```python
from build123d import *

# Parameters (mm, degrees)
SKETCH046_R     = 2.5
PAD023_DEPTH    = 2.5
SKETCH047_R     = 5
PAD024_DEPTH    = 3
FILLET003_R     = 1.5
SKETCH049_R     = 2.5
PAD025_DEPTH    = 4
SKETCH050_R     = 1.5
POCKET026_DEPTH = 4
PAD055_DEPTH    = 0.2


with BuildPart() as part:
    # Sketch046 → Pad023 (new body)
    with BuildSketch(Plane(origin=(0, 0, 30), x_dir=(1, 0, 0), z_dir=(0, 0, -1))):
        with Locations((101, 55)):
            Circle(SKETCH046_R)
    extrude(amount=-PAD023_DEPTH)

    # Sketch047 (on Face3 of Pad023) → Pad024 (join)
    with BuildSketch(Plane.XY.offset(32.5)):
        with Locations((101, -55)):
            Circle(SKETCH047_R)
    extrude(amount=PAD024_DEPTH)

    # Fillet003
    fillet003_edges = [part.edges().sort_by_distance(p)[0] for p in [
        (96, -55, 35.5),
    ]]
    fillet(fillet003_edges, radius=FILLET003_R)

    # Sketch049 → Pad025 (join)
    with BuildSketch(Plane(origin=(0, 0, 30), x_dir=(1, 0, 0), z_dir=(0, 0, -1))):
        with Locations((101, 55)):
            Circle(SKETCH049_R)
    extrude(amount=PAD025_DEPTH)

    # Sketch050 (on Face17 of Pad025) → Pocket026 (cut)
    with BuildSketch(Plane(origin=(0, 0, 26), x_dir=(1, 0, 0), z_dir=(0, 0, -1))):
        with Locations((101, 55)):
            Circle(SKETCH050_R)
    extrude(amount=-POCKET026_DEPTH, mode=Mode.SUBTRACT)


with BuildPart() as part_1:
    # Body002 placement: moved
    add(part.part.moved(Location((75, 0, 0))))

    # Sketch089 (on Face4 of Clone) → Pad055 (new body)
    with BuildSketch(Plane(origin=(176, -55, 35.5), x_dir=(1, 0, 0), z_dir=(0, 0, 1))):
        Polygon((-3, 1), (-3, -1), (-1.5, -1), (0.5, -2.5), (0.5, 2.5), (-1.5, 1), align=None)
        with BuildLine():
            ThreePointArc((1.608436, -2.050571), (2.606129, 0), (1.608436, 2.050571))
            Line((1.608436, 2.050571), (1.129955, 1.542421))
            ThreePointArc((1.129955, -1.542421), (1.744062, 0), (1.129955, 1.542421))
            Line((1.608436, -2.050571), (1.129955, -1.542421))
        make_face()
    extrude(amount=PAD055_DEPTH)


with BuildPart() as part_2:
    # Body012 placement: moved
    add(part_1.part.moved(Location((-75, 0, 0))))


solid = part_2.part
```
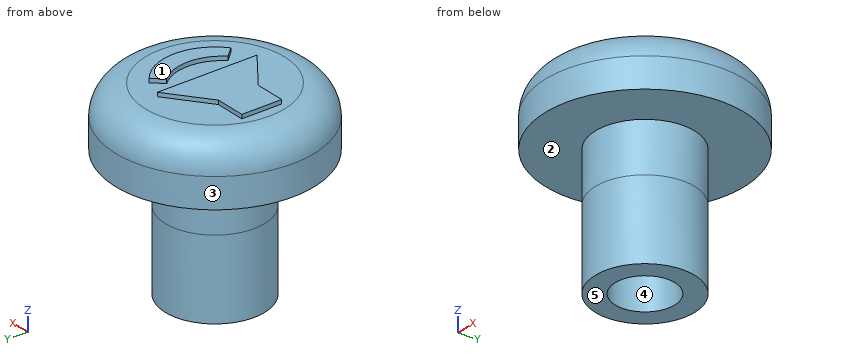
Read the model definition and answer for the solid it produces. Units are mm, in the model's axes. Face numbers are marked on the shaded views. A direction names the side the tool comes from. Round coordinates to 2 decimals unless told otherwise and drop trailing zeros. Write each loop counter-clockwise with the first axis right and the second up, starting at its lowest first coordinate (ties: lowest second). Pieces come first, ordered by that corner, then holes. Notation, with made-up numbers: (55, 19.5) -> (83, 19.5) arc R30 ccw to (83, 55.5) -> close; hole circle Ø5 at (-15, -8). An arc over 180 degrees is marked (long way). Answer in a Markdown table with one row per item. Add a question column.
1) Determine the mould class of the marked faces 3, 4 and 5 for opening direction X: pulls with the +X half, pulls with the -X half, needs draft (parallel to the pull), parting line crosses it, or undercut.
2) Find section C-C, the plane x = 101. Determine the outline of the cut face in (y, z) (3 decimals).
3) Which of the six approach directions +Z, -Z, +X, -X, +Y, -Y give full straight-line access (tool end or side, diameter ignored) to the marked faces 1 and 2?
4) Given P1, Ø2, axis at x = 99.5, y = -58, coming from the +Z side; P2, Ø1, axis at x = 101.5, y = -55.5, coming from the -Z side; P3, Ø5, axis at x = 97, z = 32, coming from the -Y side, each flat-ended and moving along its own axis, determine where each tip first touches the part or whether it passes through.
5) Find section B-B, the plane z = 28.75. Determine the outline of the cut face in (x, y), and give its area (3 significant figures).
6) Consider line 1 (Y direction, x = 101, z = 28.6); line 2 (X direction, y = -55, z = 27.2); line 3 (Z direction, x = 100.75, y = -56). Determine where each line is inside the solid, lowest interval first.
7) Find section A-A, the plane y = -55. Determine the outline of the cut face in (x, z).
Findings below:
| question | item | result |
|---|---|---|
| 1 | face 3 | parting line crosses it |
| 1 | face 4 | undercut |
| 1 | face 5 | needs draft |
| 2 | outline | (-60, 32.5) -> (-57.5, 32.5) -> (-57.5, 26) -> (-56.5, 26) -> (-56.5, 30) -> (-53.5, 30) -> (-53.5, 26) -> (-52.5, 26) -> (-52.5, 32.5) -> (-50, 32.5) -> (-50, 34) arc R1.5 ccw to (-51.5, 35.5) -> (-52.875, 35.5) -> (-52.875, 35.7) -> (-57.125, 35.7) -> (-57.125, 35.5) -> (-58.5, 35.5) arc R1.5 ccw to (-60, 34) -> close |
| 3 | face 1 | +Z, +X, -X, +Y, -Y |
| 3 | face 2 | -Z |
| 4 | P1 | z = 35.5 |
| 4 | P2 | z = 30 |
| 4 | P3 | y = -59.75 |
| 5 | outline | circle Ø5 at (101, -55); hole circle Ø3 at (101, -55) |
| 5 | area | 12.6 mm² |
| 6 | line 1 | -57.5 to -56.5, -53.5 to -52.5 |
| 6 | line 2 | 98.5 to 99.5, 102.5 to 103.5 |
| 6 | line 3 | 30 to 35.7 |
| 7 | outline | (96, 32.5) -> (98.5, 32.5) -> (98.5, 26) -> (99.5, 26) -> (99.5, 30) -> (102.5, 30) -> (102.5, 26) -> (103.5, 26) -> (103.5, 32.5) -> (106, 32.5) -> (106, 34) arc R1.5 ccw to (104.5, 35.5) -> (103.61, 35.5) -> (103.61, 35.7) -> (102.74, 35.7) -> (102.74, 35.5) -> (101.5, 35.5) -> (101.5, 35.7) -> (98, 35.7) -> (98, 35.5) -> (97.5, 35.5) arc R1.5 ccw to (96, 34) -> close |
